Input: part model. Units: mm. Frame: model coordinates. A direction names the side the tool comes from. Give positions to 0.01 mm unless a question says otherwise; leave off trailing zeros. Loops run counter-clockwise (first coordinate to the right, second up) from the corner with the lowest first, then second, coordinate; pieces in that order, holes last. Notation, with made-up numbers: M 43.5,-15.75 L 69.5,-15.75 A13 cw 69.5,2.25 Z; hole C -20.5,10.5 d10. An arc over 180 degrees is marked long. Answer as a JSON object with one key per item and string values. Group by question number.
1) Ray query, L1, parallel to Z at x = 156, y = 21.5; L2, parallel to X at y = 5.6, z = 150; L3, parallel to X at y = 1, z = 150. Return the intervals inside material, ascending.
2) Section query A-A on z = 72.5. Return loops of the section in (x, y), plus the area to 3 significant figures.
3) Draft query along X for faces 1 (the flat face through (158, 8, 8)), 2 (the flat face through (158, 19, 150)). Return one class per face: +X half, -X half, draft (parallel to the pull), parting line (faces both ways), or undercut.
4) First-contact query: P1, Ø6, axis at x = 114, z = 102, coming from the +Y side; P2, Ø8, axis at y = 27, z = 21, coming from the -X side; P3, Ø12, axis at x = 10.5, y = 20, coming from the -Z side; P4, Ø2.5, axis at x = 116.5, z = 149, coming from the -Y side. Flat tips, straight axial feed; report the tip coordinate or a pass-through.
5) Access query for faces 3 (the cylindrical face through (117.85, 1.48, 152.11)), 4 (the flat face through (158, 19, 15)), 5 (the flat face through (2.256, 19, 7)), 6 (the flat face through (15.256, 19, 7)). Directions: +Z, -Z, +X, -X, +Y, -Y. A direction counts if a zero-diameter tool reaches every point of the face in a straight line with its end or side. Return the directions, or none.
6) Section query B-B on x = 82.5. Return loops of the section in (y, z), plus the area to 3 significant figures.
Autodesk Inventor part; units mm, degrees
ref_plane "YZ Plane" through (0, 0, 0) normal (1, 0, 0) x (0, 1, 0)
ref_plane "XZ Plane" through (0, 0, 0) normal (0, 1, 0) x (-1, 0, 0)
ref_plane "XY Plane" through (0, 0, 0) normal (0, 0, 1) x (1, 0, 0)
sketch "Sketch1" plane through (0, 0, 0) normal (0, 1, 0) x (-1, 0, 0)
  line L0 (-0.256, 0) -> (-165.256, 0)
  line L1 (-165.256, 0) -> (-165.256, 165)
  line L2 (-165.256, 165) -> (-0.256, 165)
  line L3 (-0.256, 165) -> (-0.256, 0)
  point P0 (0, 0)
  dimension "d0" = 165
  dimension "d1" = 165
extrude "Extrusion1" add sketch "Sketch1" along normal blind 8
sketch "Sketch2" plane through (0, 8, 0) normal (0, 1, 0) x (1, 0, 0)
  line L0 (165.256, 0) -> (0.256, 0)
  line L1 (0.256, 0) -> (15.256, 0)
  line L2 (15.256, 0) -> (15.256, -15)
  line L3 (15.256, -15) -> (0.256, -15)
  line L4 (0.256, -15) -> (0.256, 0)
  line L5 (0.256, -165) -> (165.256, -165)
  line L6 (0.256, -165) -> (15.256, -165)
  line L7 (15.256, -165) -> (15.256, -150)
  line L8 (15.256, -150) -> (0.256, -150)
  line L9 (0.256, -150) -> (0.256, -165)
  line L10 (2.256, -152) -> (13.256, -152)
  line L11 (13.256, -152) -> (13.256, -163)
  line L12 (13.256, -163) -> (2.256, -163)
  line L13 (2.256, -163) -> (2.256, -152)
  line L14 (13.256, -13) -> (13.256, -2)
  line L15 (13.256, -2) -> (2.256, -2)
  line L16 (2.256, -2) -> (2.256, -13)
  line L17 (2.256, -13) -> (13.256, -13)
  line L18 (82.756, 0) -> (82.756, -165)
  line L19 (0.256, 0) -> (165.256, 0)
  line L20 (150.256, 0) -> (150.256, -15)
  line L21 (150.256, -15) -> (165.256, -15)
  line L22 (165.256, -15) -> (165.256, 0)
  line L23 (165.256, -165) -> (0.256, -165)
  line L24 (165.256, -165) -> (150.256, -165)
  line L25 (150.256, -165) -> (150.256, -150)
  line L26 (150.256, -150) -> (165.256, -150)
  line L27 (165.256, -150) -> (165.256, -165)
  line L28 (163.256, -152) -> (152.256, -152)
  line L29 (152.256, -152) -> (152.256, -163)
  line L30 (152.256, -163) -> (163.256, -163)
  line L31 (163.256, -163) -> (163.256, -152)
  line L32 (152.256, -13) -> (152.256, -2)
  line L33 (152.256, -2) -> (163.256, -2)
  line L34 (163.256, -2) -> (163.256, -13)
  line L35 (163.256, -13) -> (152.256, -13)
  point P0 (0, 0)
  dimension "d4" = 15
  dimension "d5" = 15
  dimension "d6" = 15
  dimension "d7" = 15
  dimension "d8" = 2
  dimension "d9" = 2
extrude "Extrusion2" add sketch "Sketch2" along normal blind 23
sketch "Sketch3" plane through (0, 8, 0) normal (0, 1, 0) x (1, 0, 0)
  line L0 (150.256, -150) -> (150.256, -165)
  line L1 (0.256, -150) -> (15.256, -150)
  line L2 (150.256, -150) -> (15.256, -150)
  line L3 (0.256, -165) -> (165.256, -165)
  line L4 (82.756, -165) -> (82.756, -150)
  line L5 (82.756, -150) -> (150.256, -150)
  circle A0 centre (116.506, -150) radius 1.6
  point P0 (0, 0)
  dimension "d12" = 3.2
extrude "Extrusion3" cut sketch "Sketch3" against normal blind 8 contours A0 L2 | L2 A0
sketch "Sketch4" plane through (0, 0, 0) normal (0, -1, 0) x (1, 0, 0)
  circle A0 centre (116.506, 150) radius 1.6
  circle A1 centre (116.506, 150) radius 2.5
  point P0 (0, 0)
  dimension "d15" = 5
extrude "Extrusion4" cut sketch "Sketch4" against normal blind 3
properties part number "piano inferiore"
Output:
{
 "1": {"L1": "z = 0 to 2, 13 to 15, 150 to 152, 163 to 165", "L2": "x = 0.26 to 114.91, 118.11 to 165.26", "L3": "x = 0.26 to 114.01, 119.01 to 165.26"},
 "2": {"outline": "M 0.26,0 L 165.26,0 L 165.26,8 L 0.26,8 Z", "area": "1,320 mm^2"},
 "3": {"face 1": "undercut", "face 2": "draft"},
 "4": {"P1": "stops at y = 8", "P2": "passes through", "P3": "stops at z = 0", "P4": "stops at y = 3"},
 "5": {"face 3": "-Y", "face 4": "+X, -X, +Y", "face 5": "+Y", "face 6": "+Z, -Z, +Y"},
 "6": {"outline": "M 0,0 L 8,0 L 8,165 L 0,165 Z", "area": "1,320 mm^2"}
}
